The model under review builds one solid part; all positions refer to its coordinate system, in mm. Round coordinates to 2 decimals unless told otherwise and drop trailing zeros. Loops run counter-clockwise (first coordinate to the right, second up) from the corner with the lowest first, then second, coordinate; pieces in that order, holes last. Notation, with made-up numbers: (77.25, 51.5) -> (92.25, 51.5) arc R36 ccw to (92.25, 86.5) -> close; hole circle Ø4 at (4, 43.25). An arc over 180 degrees is marked (long way). Write each question's results on one line, items separated by ' | '. Start each with the question number.
Item 1: We need section B-B (z = 13.5). Give the boundary of the cut face in (x, y), and give its area (3 significant figures).
Item 2: We need section C-C (y = 0.8). Give the number of separate pieces and of enclosed holes in the cut face, and give its area (3 significant figures).
Item 3: Clearance check with flat-ended pins moving along their axes: pin 1 Ø5 at (x, z) = (-44, -5) entering from -Y; pin 2 Ø1.2 at (y, z) = (2.5, 4) entering from -X. State where each tip first meets the part, or that it passes through.
Item 4: We need section A-A (x = -101). Give the boundary of the cut face in (y, z).
Item 5: For L1, parallel to X at y = 2.4, z = 8; L2, parallel to X at y = 1.6, z = 144; L3, parallel to X at y = 2, z = 176, list the stretches that pass through material, from the lowest coordinate up. Write a range as from..to.
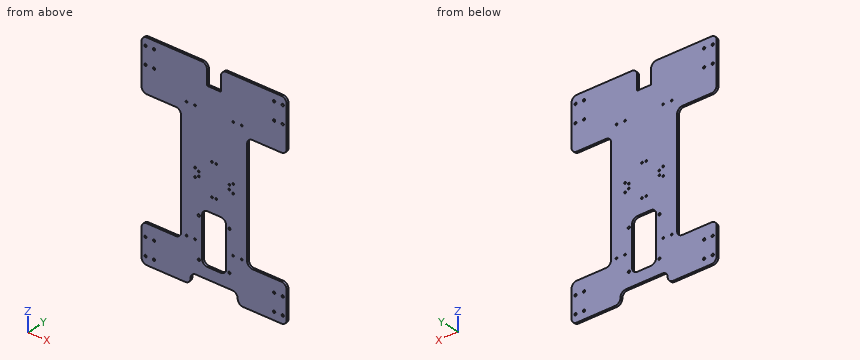
from build123d import *

# Parameters (mm, degrees)
SKETCH_1_W           = 271
SKETCH_1_H           = 381
EXTRUDE_2_DEPTH      = 4
SKETCH_4_R           = 2.1
CUT_EXTRUDE_3_DEPTH  = 4
SKETCH_5_W           = 26
SKETCH_5_H           = 74.1
CUT_EXTRUDE_4_DEPTH  = 4
SKETCH_6_W           = 148
SKETCH_6_H           = 216
CUT_EXTRUDE_6_DEPTH  = 4
SKETCH_7_R           = 1.6
CUT_EXTRUDE_7_DEPTH  = 4
SKETCH_8_R           = 1.6
CUT_EXTRUDE_8_DEPTH  = 4
SKETCH_9_W           = 45
SKETCH_9_H           = 93.3
CUT_EXTRUDE_9_DEPTH  = 4
SKETCH_10_R          = 2.1
CUT_EXTRUDE_10_DEPTH = 4
SKETCH_11_R          = 1.6
CUT_EXTRUDE_11_DEPTH = 4
SKETCH_12_R          = 2.1
CUT_EXTRUDE_12_DEPTH = 4
SKETCH_13_W          = 88
SKETCH_13_H          = 40
CUT_EXTRUDE_13_DEPTH = 4
FILLET_3_R           = 10
FILLET_5_R           = 10
FILLET_6_R           = 1
SKETCH_15_R          = 1.6
CUT_EXTRUDE_17_DEPTH = 10


with BuildPart() as part:
    # 草图1 → 凸台-拉伸2 (new body)
    with BuildSketch(Plane(origin=(0, 0, 0), x_dir=(1, 0, 0), z_dir=(0, 1, 0))):
        Rectangle(SKETCH_1_W, SKETCH_1_H)
    extrude(amount=EXTRUDE_2_DEPTH)

    # 草图4 → 切除-拉伸3 (cut)
    with BuildSketch(Plane(origin=(0, 4, 0), x_dir=(1, 0, 0), z_dir=(0, 1, 0))):
        with Locations(Location((-128, -176, 0), (0, 0, 270))):
            Circle(SKETCH_4_R)
        with Locations(Location((-128, -144, 0), (0, 0, 270))):
            Circle(SKETCH_4_R)
        with Locations(Location((-112, -144, 0), (0, 0, 270))):
            Circle(SKETCH_4_R)
        with Locations(Location((-112, -176, 0), (0, 0, 270))):
            Circle(SKETCH_4_R)
        with Locations(Location((112, -144, 0), (0, 0, 90))):
            Circle(SKETCH_4_R)
        with Locations(Location((128, -144, 0), (0, 0, 90))):
            Circle(SKETCH_4_R)
        with Locations(Location((128, -176, 0), (0, 0, 90))):
            Circle(SKETCH_4_R)
        with Locations(Location((112, -176, 0), (0, 0, 90))):
            Circle(SKETCH_4_R)
        with Locations(Location((112, 176, 0), (0, 0, 270))):
            Circle(SKETCH_4_R)
        with Locations(Location((128, 176, 0), (0, 0, 270))):
            Circle(SKETCH_4_R)
        with Locations(Location((128, 144, 0), (0, 0, 270))):
            Circle(SKETCH_4_R)
        with Locations(Location((112, 144, 0), (0, 0, 270))):
            Circle(SKETCH_4_R)
        with Locations(Location((-112, 176, 0), (0, 0, 90))):
            Circle(SKETCH_4_R)
        with Locations(Location((-112, 144, 0), (0, 0, 90))):
            Circle(SKETCH_4_R)
        with Locations(Location((-128, 144, 0), (0, 0, 90))):
            Circle(SKETCH_4_R)
        with Locations(Location((-128, 176, 0), (0, 0, 90))):
            Circle(SKETCH_4_R)
    extrude(amount=-CUT_EXTRUDE_3_DEPTH, mode=Mode.SUBTRACT)

    # 草图5 → 切除-拉伸4 (cut)
    with BuildSketch(Plane(origin=(0, 4, 0), x_dir=(1, 0, 0), z_dir=(0, 1, 0))):
        with Locations((0, -190.5)):
            Rectangle(SKETCH_5_W, SKETCH_5_H)
    extrude(amount=-CUT_EXTRUDE_4_DEPTH, mode=Mode.SUBTRACT)

    # 草图6 → 切除-拉伸6 (cut)
    with BuildSketch(Plane(origin=(0, 4, 0), x_dir=(1, 0, 0), z_dir=(0, 1, 0))):
        with Locations((135.5, 12.5)):
            Rectangle(SKETCH_6_W, SKETCH_6_H)
        with Locations((-135.5, 12.5)):
            Rectangle(SKETCH_6_W, SKETCH_6_H)
    extrude(amount=-CUT_EXTRUDE_6_DEPTH, mode=Mode.SUBTRACT)

    # 草图7 → 切除-拉伸7 (cut)
    with BuildSketch(Plane(origin=(0, 4, 0), x_dir=(1, 0, 0), z_dir=(0, 1, 0))):
        with Locations(Location((-51.5, -112, 0), (0, 0, 270))):
            Circle(SKETCH_7_R)
        with Locations(Location((-35.5, -112, 0), (0, 0, 270))):
            Circle(SKETCH_7_R)
        with Locations(Location((35.5, -112, 0), (0, 0, 90))):
            Circle(SKETCH_7_R)
        with Locations(Location((51.5, -112, 0), (0, 0, 90))):
            Circle(SKETCH_7_R)
    extrude(amount=-CUT_EXTRUDE_7_DEPTH, mode=Mode.SUBTRACT)

    # 草图8 → 切除-拉伸8 (cut)
    with BuildSketch(Plane(origin=(0, 4, 0), x_dir=(1, 0, 0), z_dir=(0, 1, 0))):
        with Locations(Location((-35.5, 8, 0), (0, 0, 270))):
            Circle(SKETCH_8_R)
        with Locations(Location((-35.5, -8, 0), (0, 0, 270))):
            Circle(SKETCH_8_R)
        with Locations(Location((35.5, -8, 0), (0, 0, 90))):
            Circle(SKETCH_8_R)
        with Locations(Location((35.5, 8, 0), (0, 0, 90))):
            Circle(SKETCH_8_R)
    extrude(amount=-CUT_EXTRUDE_8_DEPTH, mode=Mode.SUBTRACT)

    # 草图9 → 切除-拉伸9 (cut)
    with BuildSketch(Plane(origin=(0, 4, 0), x_dir=(1, 0, 0), z_dir=(0, 1, 0))):
        with Locations((0, 102.85)):
            Rectangle(SKETCH_9_W, SKETCH_9_H)
    extrude(amount=-CUT_EXTRUDE_9_DEPTH, mode=Mode.SUBTRACT)

    # 草图10 → 切除-拉伸10 (cut)
    with BuildSketch(Plane(origin=(0, 4, 0), x_dir=(1, 0, 0), z_dir=(0, 1, 0))):
        with Locations(Location((-28.5, 69.5, 0), (0, 0, 270))):
            Circle(SKETCH_10_R)
        with Locations(Location((28.5, 69.5, 0), (0, 0, 90))):
            Circle(SKETCH_10_R)
    extrude(amount=-CUT_EXTRUDE_10_DEPTH, mode=Mode.SUBTRACT)

    # 草图11 → 切除-拉伸11 (cut)
    with BuildSketch(Plane(origin=(0, 4, 0), x_dir=(1, 0, 0), z_dir=(0, 1, 0))):
        with Locations(Location((-51.5, 112, 0), (0, 0, 270))):
            Circle(SKETCH_11_R)
        with Locations(Location((-35.5, 112, 0), (0, 0, 270))):
            Circle(SKETCH_11_R)
        with Locations(Location((35.5, 112, 0), (0, 0, 90))):
            Circle(SKETCH_11_R)
        with Locations(Location((51.5, 112, 0), (0, 0, 90))):
            Circle(SKETCH_11_R)
    extrude(amount=-CUT_EXTRUDE_11_DEPTH, mode=Mode.SUBTRACT)

    # 草图12 → 切除-拉伸12 (cut)
    with BuildSketch(Plane(origin=(0, 4, 0), x_dir=(1, 0, 0), z_dir=(0, 1, 0))):
        with Locations(Location((-28.5, 143.5, 0), (0, 0, 270))):
            Circle(SKETCH_12_R)
        with Locations(Location((28.5, 143.5, 0), (0, 0, 90))):
            Circle(SKETCH_12_R)
    extrude(amount=-CUT_EXTRUDE_12_DEPTH, mode=Mode.SUBTRACT)

    # 草图13 → 切除-拉伸13 (cut)
    with BuildSketch(Plane(origin=(0, 4, 0), x_dir=(1, 0, 0), z_dir=(0, 1, 0))):
        with Locations((0, 190.5)):
            Rectangle(SKETCH_13_W, SKETCH_13_H)
    extrude(amount=-CUT_EXTRUDE_13_DEPTH, mode=Mode.SUBTRACT)

    # 圆角3
    fillet_3_edges = [part.edges().sort_by_distance(p)[0] for p in [
        (22.5, 2, -149.5),
        (22.5, 2, -56.2),
        (-22.5, 2, -56.2),
        (-22.5, 2, -149.5),
    ]]
    fillet(fillet_3_edges, radius=FILLET_3_R)

    # 圆角5
    fillet_5_edges = [part.edges().sort_by_distance(p)[0] for p in [
        (-44, 2, -170.5),
        (-44, 2, -190.5),
        (-135.5, 2, -190.5),
        (-135.5, 2, -120.5),
        (-61.5, 2, -120.5),
        (-61.5, 2, 95.5),
        (-135.5, 2, 95.5),
        (-135.5, 2, 190.5),
        (-13, 2, 190.5),
        (13, 2, 190.5),
        (135.5, 2, 190.5),
        (135.5, 2, 95.5),
        (61.5, 2, 95.5),
        (61.5, 2, -120.5),
        (135.5, 2, -120.5),
        (135.5, 2, -190.5),
        (44, 2, -190.5),
        (44, 2, -170.5),
    ]]
    fillet(fillet_5_edges, radius=FILLET_5_R - 0.0001)  # a hair under: the kernel refuses the full size

    # 圆角6
    fillet_6_edges = [part.edges().sort_by_distance(p)[0] for p in [
        (13, 2, 153.45),
        (-13, 2, 153.45),
    ]]
    fillet(fillet_6_edges, radius=FILLET_6_R)

    # 草图15 → 切除-拉伸17 (cut)
    with BuildSketch(Plane(origin=(0, 4, 0), x_dir=(1, 0, 0), z_dir=(0, 1, 0))):
        with Locations(Location((-28.5, -4, 0), (0, 0, 270))):
            Circle(SKETCH_15_R)
        with Locations(Location((-28.5, 4, 0), (0, 0, 270))):
            Circle(SKETCH_15_R)
        with Locations(Location((-4, 29.5, 0), (0, 0, 270))):
            Circle(SKETCH_15_R)
        with Locations(Location((28.5, 4, 0), (0, 0, 270))):
            Circle(SKETCH_15_R)
        with Locations(Location((28.5, -4, 0), (0, 0, 270))):
            Circle(SKETCH_15_R)
        with Locations(Location((4, 29.5, 0), (0, 0, 270))):
            Circle(SKETCH_15_R)
        with Locations(Location((4, -29.5, 0), (0, 0, 270))):
            Circle(SKETCH_15_R)
        with Locations(Location((-4, -29.5, 0), (0, 0, 270))):
            Circle(SKETCH_15_R)
    extrude(amount=-CUT_EXTRUDE_17_DEPTH, mode=Mode.SUBTRACT)


solid = part.part
Here are the results:
1) outline: (-61.5, 0) -> (61.5, 0) -> (61.5, 4) -> (-61.5, 4) -> close | area: 492 mm2
2) separate pieces: 1 | enclosed holes: 41 | area: 63,900 mm2
3) pin 1: stops at y = 0 | pin 2: stops at x = -61.5
4) outline: (0, -190.5) -> (4, -190.5) -> (4, -120.5) -> (0, -120.5) -> close; (0, 95.5) -> (4, 95.5) -> (4, 190.5) -> (0, 190.5) -> close
5) L1: x = -61.5..-37.1, -33.9..33.9, 37.1..61.5 | L2: x = -135.5..-130.1, -125.9..-114.1, -109.9..109.9, 114.1..125.9, 130.1..135.5 | L3: x = -135.5..-130.1, -125.9..-114.1, -109.9..-13, 13..109.9, 114.1..125.9, 130.1..135.5
